Source: CAD feature listing. Evaluate the final solid. Frame: model axes, mm. A direction names the side the tool comes from. Give positions to 0.01 mm unless a question says otherwise; leave off trailing zeros. Order: outer loops, then holes, each group sorted by start corner. A loop starts at its lowest first (then second) coordinate and runs counter-clockwise, first axis right, second up. Notation, with made-up numbers: M -30.75,75 L -24.75,75 A8 ccw -24.75,84 Z; hole C 29,-24 d9. An arc over 180 degrees is marked long. Return JSON: item names as keys, results as strings.
Autodesk Inventor part; units mm, degrees
ref_plane "우측면도" through (0, 0, 0) normal (1, 0, 0) x (0, 1, 0)
ref_plane "평면도" through (0, 0, 0) normal (0, 1, 0) x (-1, 0, 0)
ref_plane "정면도" through (0, 0, 0) normal (0, 0, 1) x (1, 0, 0)
sketch "스케치1" plane through (0, 0, 0) normal (0, 1, 0) x (-1, 0, 0)
  line L0 (0, 0) -> (0, -100)
  line L1 (0, -100) -> (-50, -100)
  line L2 (-50, -100) -> (-50, 0)
  line L3 (-50, 0) -> (0, 0)
  line L4 (2.5, -102.5) -> (2.5, 2.5)
  line L5 (2.5, 2.5) -> (-52.5, 2.5)
  line L6 (-52.5, 2.5) -> (-52.5, -102.5)
  line L7 (-52.5, -102.5) -> (2.5, -102.5)
  line L8 (1, -101) -> (1, 1)
  line L9 (1, 1) -> (-51, 1)
  line L10 (-51, 1) -> (-51, -101)
  line L11 (-51, -101) -> (1, -101)
  line L12 (1.5, -101.5) -> (1.5, 1.5)
  line L13 (1.5, 1.5) -> (-51.5, 1.5)
  line L14 (-51.5, 1.5) -> (-51.5, -101.5)
  line L15 (-51.5, -101.5) -> (1.5, -101.5)
  dimension "d0" = 50
  dimension "d1" = 100
  dimension "d2" = 2.5
  dimension "d3" = 1.5
  dimension "d4" = 0.5
extrude "돌출1" add sketch "스케치1" along normal blind 1 contours L0 L1 L2 L3 | L7 L6 L5 L4 | L11 L10 L9 L8 | L15 L14 L13 L12
sketch "스케치2" plane through (0, 1, 0) normal (0, 1, 0) x (1, 0, 0)
  line L0 (51.5, -1.5) -> (51.5, 101.5)
  line L1 (51, -1) -> (51, 101)
  line L2 (51.5, 101.5) -> (-1.5, 101.5)
  line L3 (51, 101) -> (-1, 101)
  line L4 (-1.5, 101.5) -> (-1.5, -1.5)
  line L5 (-1, 101) -> (-1, -1)
  line L6 (-1, -1) -> (51, -1)
  line L7 (-1.5, -1.5) -> (51.5, -1.5)
  point P0 (0, 0)
extrude "돌출3" add sketch "스케치2" along normal blind 2.5
properties part number "호출벨 new 커버"
1. Set-up query: faces 1 (the face through (25, 2, 1.5)), 2 (the face through (-1.5, 2, -51)), 3 (the face through (51.5, 2, -49)), 4 (the face through (25, 0, -49)), 5 (the face through (51, 2, -49)). Return all of +Z, -Z, +X, -X, +Y, -Y with unobstructed straight access to the full face (end or side cutting, diameter ignored); none if empty.
Evaluation:
{"face 1": "+Z, +X, -X, +Y", "face 2": "+Z, -Z, -X, +Y", "face 3": "+Z, -Z, +X, +Y", "face 4": "+Z, -Z, +X, -X, -Y", "face 5": "+Y"}
2. Ray query, probe 1 along X at (y, z) = (1.2, -73.5); probe 2 along Z at (x, y) = (12.5, 2.1); probe 3 along Y at (x, z) = (16, -84). Return the intervals inside material, ascending.
Evaluation:
{"probe 1": "x = -1.5 to -1, 51 to 51.5", "probe 2": "z = -101.5 to -101, 1 to 1.5", "probe 3": "y = 0 to 1"}
3. First-contact query: pin 1 (2 mm diameter, centred on x = 44.5, z = -75, fed in from +Y); pin 2 (0.8 mm diameter, centred on x = 24.5, y = 2.5, fed in from +Z); pin 3 (3 mm diameter, centred on x = 46.5, z = -22, fed in from -Y); pin 4 (0.8 mm diameter, centred on x = 16, y = 2, fed in from -Z). Flat tips, straight axial feed; report the tip coordinate or a pass-through.
Evaluation:
{"pin 1": "stops at y = 1", "pin 2": "stops at z = 1.5", "pin 3": "stops at y = 0", "pin 4": "stops at z = -101.5"}
4. Section query A-A (y = 1.9). Return loops of the section in (x, z), then the cut area to 3 significant figures.
Evaluation:
{"outline": "M -1.5,-101.5 L 51.5,-101.5 L 51.5,1.5 L -1.5,1.5 Z; hole M -1,-101 L 51,-101 L 51,1 L -1,1 Z", "area": "155 mm^2"}
5. Section query B-B (x = 40). Return loops of the section in (y, z), then the cut area to 4 significant figures.
Evaluation:
{"outline": "M 0,-102.5 L 1,-102.5 L 1,-101.5 L 3.5,-101.5 L 3.5,-101 L 1,-101 L 1,1 L 3.5,1 L 3.5,1.5 L 1,1.5 L 1,2.5 L 0,2.5 Z", "area": "107.5 mm^2"}
6. Draft query along Z for faces 6 (the face through (52, 1, -50)), 7 (the face through (25, 2, -101)), 8 (the face through (-1, 2, -51)), 9 (the face through (25, 2, -101.5)). Return one class per face: pulls with the +Z half, pulls with the -Z half, needs draft (parallel to the pull), parting line crosses it, or undercut.
Evaluation:
{"face 6": "needs draft", "face 7": "undercut", "face 8": "undercut", "face 9": "pulls with the -Z half"}
7. Section query C-C (z = -38.5). Return loops of the section in (x, y), then the cut area to 3 significant figures.
Evaluation:
{"outline": "M -2.5,0 L 52.5,0 L 52.5,1 L 51.5,1 L 51.5,3.5 L 51,3.5 L 51,1 L -1,1 L -1,3.5 L -1.5,3.5 L -1.5,1 L -2.5,1 Z", "area": "57.5 mm^2"}
